Geometry: see drawing. Coordinates: mm, zero at the bounding-box minimum. A direction names the side the tool comes from. Give positions to 0.01 mm unless a question says otherwise; leave off trailing zeros. Write each loop counter-clockwise with the first axis right and the second up, starting at its lowest first coordinate (ties: lowest second). Pieces come first, ordered by that corner, then holes. Notation, with made-up numbers: (55.25, -6) -> (93.25, -6) arc R26 ccw to (93.25, 11) -> close; hole circle Ø7 at (-10.5, 49.25). An arc over 180 degrees is marked (long way). Answer as a JSON object with one key per item and string values. Group by question number.
Item 1: Section query B-B on y = 16. Give the number of separate pieces and of enclosed holes in the cut face, plus the area to 3 significant figures.
Item 2: Access query for the marked faces 5, 6, 7 and 8. Directions: +Z, -Z, +X, -X, +Y, -Y. A direction counts if a zero-diameter tool reaches every point of the face in a straight line with its end or side. Return the directions, or none.
Item 3: Pull-direction query (Z, two-part tool) for the marked faces 1, 2, 3 and 4; classes: pulls with the +Z half, pulls with the -Z half, needs draft (parallel to the pull), parting line crosses it, or undercut.
Item 4: Section query D-D on z = 37. Return the cut outline in (x, y), plus the area to 3 significant figures.
Item 5: Ray query, probe 1 along X at (y, z) = (29, 33); probe 2 along Z at (x, y) = (33, 16); probe 3 along X at (y, z) = (23.5, 9.5). Return the intervals inside material, ascending. Write a range as from..to.
Item 6: Section query C-C on x = 87. Return the cut outline in (y, z), plus the area to 3 significant figures.
Item 7: Section query A-A on z = 46. Return the cut outline in (x, y), plus the area to 3 significant figures.
Item 8: First-contact query: pin 1 Ø4 at (y, z) = (3.5, 19.5) entering from +X; pin 2 Ø17 at (y, z) = (16, 46) entering from -X; pin 3 Ø8 at (x, y) = (34, 27.5) entering from +Z. Flat tips, straight axial feed; report the tip coordinate or a pass-through.
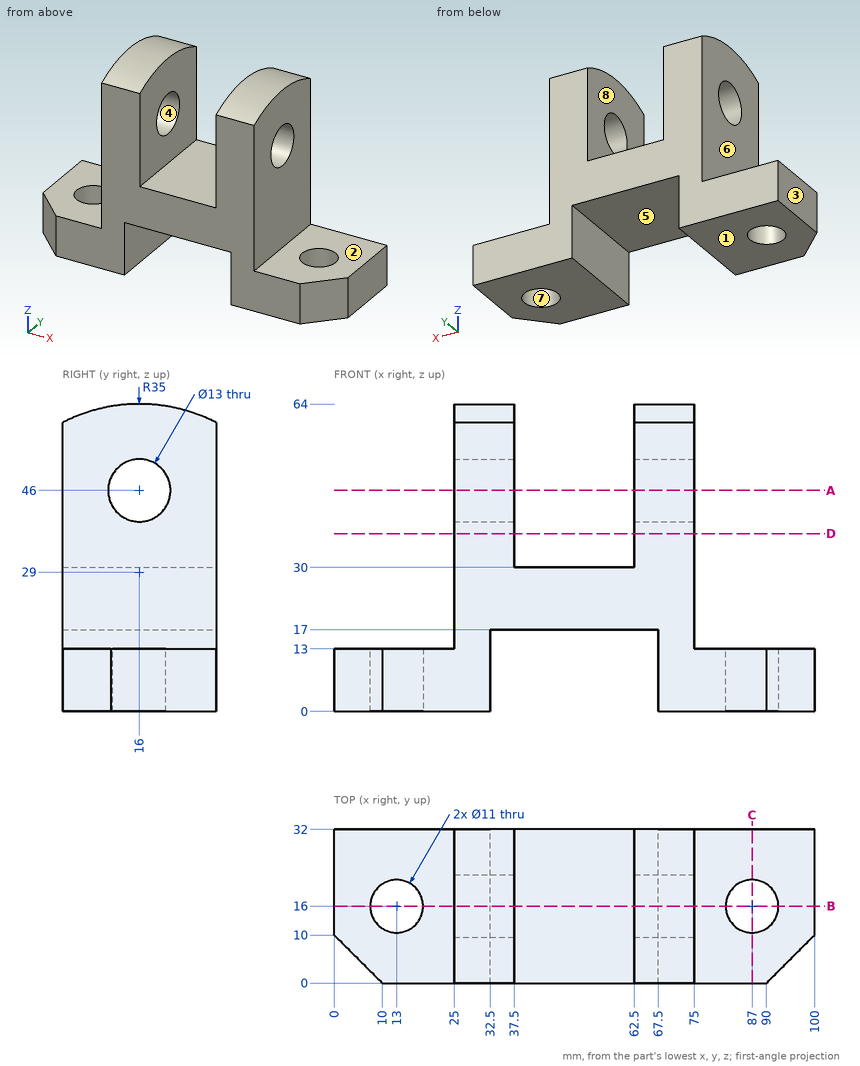
Worked answers:
{
 "1": {"separate pieces": "5", "enclosed holes": "0", "area": "1,790 mm^2"},
 "2": {"face 5": "-Z, +Y, -Y", "face 6": "+Z, -X, +Y, -Y", "face 7": "+Z, -Z", "face 8": "+Z, +Y, -Y"},
 "3": {"face 1": "pulls with the -Z half", "face 2": "pulls with the +Z half", "face 3": "needs draft", "face 4": "undercut"},
 "4": {"outline": "(25, 0) -> (37.5, 0) -> (37.5, 32) -> (25, 32) -> close; (62.5, 0) -> (75, 0) -> (75, 32) -> (62.5, 32) -> close", "area": "800 mm^2"},
 "5": {"probe 1": "25..37.5, 62.5..75", "probe 2": "17..39.5, 52.5..64", "probe 3": "0..32.5, 67.5..100"},
 "6": {"outline": "(0, 0) -> (10.5, 0) -> (10.5, 13) -> (0, 13) -> close; (21.5, 0) -> (32, 0) -> (32, 13) -> (21.5, 13) -> close", "area": "273 mm^2"},
 "7": {"outline": "(25, 0) -> (37.5, 0) -> (37.5, 9.5) -> (25, 9.5) -> close; (25, 22.5) -> (37.5, 22.5) -> (37.5, 32) -> (25, 32) -> close; (62.5, 0) -> (75, 0) -> (75, 9.5) -> (62.5, 9.5) -> close; (62.5, 22.5) -> (75, 22.5) -> (75, 32) -> (62.5, 32) -> close", "area": "475 mm^2"},
 "8": {"pin 1": "x = 75", "pin 2": "x = 25", "pin 3": "z = 63.19"}
}
